Source: CAD feature listing. Evaluate the final solid. Frame: model axes, mm. A direction names the side the tool comes from. Coordinates: 2 decimals unless noted, no trailing zeros. Write each loop counter-clockwise with the first axis right and the second up, starting at its lowest first coordinate (ties: lowest second). Pieces come first, ordered by that corner, then holes. Notation, with made-up numbers: (9, -9.75) -> (39, -9.75) arc R21 cw to (39, 5.25) -> close; hole circle Ø2 at (54, 81). An arc over 180 degrees is marked (long way). Write item = value, one per line.
from build123d import *

# Parameters (mm, degrees)
SKETCH1_R           = 1.5
SKETCH1_R_2         = 4.25
SKETCH1_R_3         = 1
BOSS_EXTRUDE2_DEPTH = 5
SKETCH2_R           = 5
CUT_EXTRUDE1_DEPTH  = 10


with BuildPart() as part:
    # Sketch1 → Boss-Extrude2 (new body)
    with BuildSketch(Plane.XY):
        with BuildLine():
            Line((45.25091594, -25.207708346), (50.00091594, -20.457708346))
            Line((50.00091594, -20.457708346), (50.00091594, 24.688738263))
            Line((50.00091594, 24.688738263), (45.147362549, 29.542291654))
            Line((45.147362549, 29.542291654), (26.35446933, 29.542291654))
            Line((26.35446933, 29.542291654), (21.25091594, 24.438738263))
            Line((21.25091594, 24.438738263), (21.25091594, 18.042291654))
            Line((21.25091594, 18.042291654), (20.408095363, 18.042291654))
            Line((20.408095363, 18.042291654), (16.70086026, 18.042291654))
            ThreePointArc((16.70086026, 18.042291654), (12.892426636, 17.542145454), (9.3422674, 16.075624987))
            ThreePointArc((9.3422674, 16.075624987), (2.182128173, 13.100539865), (-5.49908406, 12.043324729))
            Line((-5.49908406, 12.043324729), (-5.49908406, 12.039085999))
            ThreePointArc((-5.49908406, 12.039085999), (-15.49908406, 2.292291654), (-5.49908406, -7.454502691))
            Line((-5.49908406, -7.454502691), (-5.49908406, -7.458741422))
            ThreePointArc((-5.49908406, -7.458741422), (2.182128173, -8.515956557), (9.3422674, -11.491041679))
            ThreePointArc((9.3422674, -11.491041679), (12.892426636, -12.957562146), (16.70086026, -13.457708346))
            Line((16.70086026, -13.457708346), (20.408095363, -13.457708346))
            Line((20.408095363, -13.457708346), (21.25091594, -13.457708346))
            Line((21.25091594, -13.457708346), (21.25091594, -20.207708346))
            Line((21.25091594, -20.207708346), (26.25091594, -25.207708346))
            Line((26.25091594, -25.207708346), (45.25091594, -25.207708346))
        make_face()
        with Locations((46.75091594, -7.707708346)):
            Circle(SKETCH1_R, mode=Mode.SUBTRACT)
        with Locations((46.75091594, 12.292291654)):
            Circle(SKETCH1_R, mode=Mode.SUBTRACT)
        with Locations((33.50091594, 14.792291654)):
            Circle(SKETCH1_R_2, mode=Mode.SUBTRACT)
        with Locations((33.50091594, -10.207708346)):
            Circle(SKETCH1_R_2, mode=Mode.SUBTRACT)
        with Locations((19.25091594, 12.292291654)):
            Circle(SKETCH1_R, mode=Mode.SUBTRACT)
        with Locations((19.25091594, -7.707708346)):
            Circle(SKETCH1_R, mode=Mode.SUBTRACT)
        with Locations((-5.74908406, 2.292291654)):
            Circle(SKETCH1_R, mode=Mode.SUBTRACT)
        with Locations((1.25091594, 2.354746229)):
            Circle(SKETCH1_R_3, mode=Mode.SUBTRACT)
        with Locations((-0.755373293, -2.613098521)):
            Circle(SKETCH1_R_3, mode=Mode.SUBTRACT)
        with Locations((-5.686629485, -4.707708346)):
            Circle(SKETCH1_R_3, mode=Mode.SUBTRACT)
        with Locations((-10.654474236, -2.701419114)):
            Circle(SKETCH1_R_3, mode=Mode.SUBTRACT)
        with Locations((-12.74908406, 2.229837079)):
            Circle(SKETCH1_R_3, mode=Mode.SUBTRACT)
        with Locations((-10.742794828, 7.197681829)):
            Circle(SKETCH1_R_3, mode=Mode.SUBTRACT)
        with Locations((-5.811538636, 9.292291654)):
            Circle(SKETCH1_R_3, mode=Mode.SUBTRACT)
        with Locations((-0.843693885, 7.286002421)):
            Circle(SKETCH1_R_3, mode=Mode.SUBTRACT)
    extrude(amount=BOSS_EXTRUDE2_DEPTH)

    # Sketch2 → Cut-Extrude1 (cut)
    with BuildSketch(Plane.XY.offset(5)):
        with Locations((-5.74908406, 2.292291654)):
            Circle(SKETCH2_R)
    extrude(amount=-CUT_EXTRUDE1_DEPTH, mode=Mode.SUBTRACT)


solid = part.part
1) Cut plane D-D, the plane x = 15. Output: boundary loops of the cut face in (y, z), and give its area (3 significant figures).
Answer block:
outline = (-13.36, 0) -> (17.94, 0) -> (17.94, 5) -> (-13.36, 5) -> close
area = 157 mm2
2) Material intervals for probe 1 along Y at (x, z) = (-5.5, 4.75); probe 2 along Y at (x, z) = (-11, 2.1); probe 3 along Y at (x, z) = (0, 0.9), sorted ascending. Write a range as [from, to].
Answer block:
probe_1 = [-7.45, -5.69], [-3.73, -2.7], [7.29, 8.34], [10.24, 12.04]
probe_2 = [-5.92, -3.64], [-1.76, 6.23], [8.16, 10.51]
probe_3 = [-8.01, -3.27], [-1.96, 6.75], [7.82, 12.59]
3) First-contact query: pin 1 Ø2.5 at (x, y) = (46.75, 12.29) entering from +Z. Flat tip, straight axial feed; report the tip coordinate or a pass-through.
Answer block:
pin_1 = through
4) Cut plane C-C, the plane y = -19.5. Output: boundary loops of the cut face in (x, z), and give its area (3 significant figures).
Answer block:
outline = (21.25, 0) -> (50, 0) -> (50, 5) -> (21.25, 5) -> close
area = 144 mm2
5) Reachability of faces 5 (the cylindrical face through (-4.73, -4.41, 2.46)), 6 (the flat face through (19, 18.042, 2)), 7 (the flat face through (21.251, -17, 2)) from +Z, -Z, +X, -X, +Y, -Y: full face, straight path, thin tool, end or side. Return the list, or none.
Answer block:
face_5 = +Z, -Z
face_6 = +Z, -Z, -X, +Y
face_7 = +Z, -Z, -X, -Y
6) Cut plane B-B, the plane z = 1.15. Give the number of separate pieces and of enclosed holes in the cut face, and give its area (3 significant figures).
Answer block:
separate_pieces = 1
enclosed_holes = 15
area = 2,130 mm2
7) Cut plane A-A, the plane x = 37. Output: boundary loops of the cut face in (y, z), and give its area (3 significant figures).
Answer block:
outline = (-25.21, 0) -> (-12.62, 0) -> (-12.62, 5) -> (-25.21, 5) -> close; (-7.8, 0) -> (12.38, 0) -> (12.38, 5) -> (-7.8, 5) -> close; (17.2, 0) -> (29.54, 0) -> (29.54, 5) -> (17.2, 5) -> close
area = 226 mm2
8) Pull-direction query (Y, two-part tool) for faces 1 (the flat face through (21.251, 21, 2)), 2 (the cylindrical face through (2.08, -8.49, 2.46)), 3 (the cylindrical face through (48.182, 12.743, 2.465)), 4 (the cylindrical face through (-10.87, 8.19, 2.46)); classes: +Y half, -Y half, draft (parallel to the pull), parting line (faces both ways), or undercut.
Answer block:
face_1 = draft
face_2 = -Y half
face_3 = undercut
face_4 = undercut
